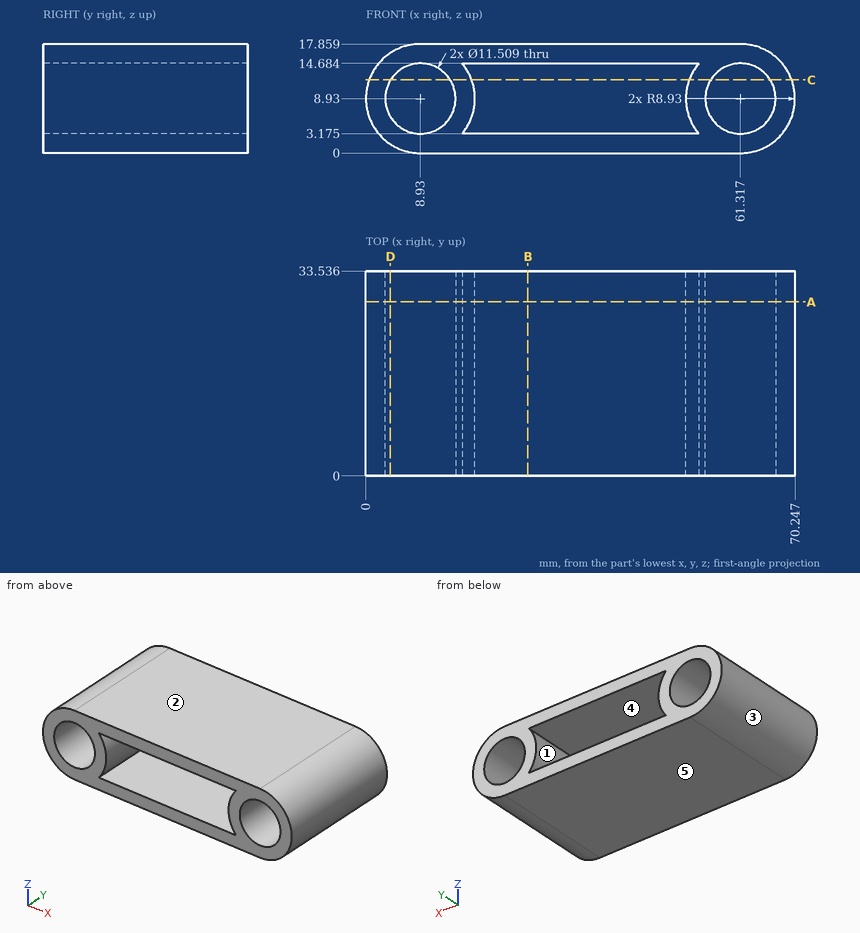
Geometry check sheet. Reference: drawing and pictorial views, mm from the part's lowest x, y, z. A direction names the side the tool comes from. Round coordinates to 2 decimals unless told otherwise and drop trailing zeros. Write each loop counter-clockwise with the first axis right and the second up, starting at its lowest first coordinate (ties: lowest second). Pieces come first, ordered by that corner, then holes.
1. Draft check along Z on the marked faces 1, 2 and 3. Enter one of: +Z half, -Z half, draft (parallel to the pull), parting line (faces both ways), or undercut.
2. Scan lines: L1, parallel to X at y = 16.5, z = 8.5 (1 decimal); L2, parallel to Z at x = 45, y = 4.5 (1 decimal); L3, parallel to X at y = 19, z = 8.75 (1 decimal). Record each from-to range of solid material in increasing order.
3. Section check C-C on z = 12. State how many separate pieces and enclosed holes the cut face has, plus the area to 3 significant figures.
4. Gauge pin test, flat ends, axial feed: P1, Ø5, axis at x = 36, z = 6.5, coming from the +Y side; P2, Ø2, axis at y = 9.5, z = 7.5, coming from the +X side; P3, Ø1.5, axis at x = 7.5, y = 13.5, coming from the +Z side. Record the tip position at first contact, or that the pin passes through.
5. Access from +Z, -Z, +X, -X, +Y, -Y to the whole of each face (thin tool, end or side, straight path). Record for the marked faces 4 and 5.
6. Section check A-A on y = 28.5. Enter the section's corners in (x, z) (1 decimal).
7. Section check D-D on x = 4. Enter the section's corners in (y, z) (1 decimal), plus the area to 3 significant figures.
8. Section check B-B on x = 26.5. Enter the section's corners in (y, z) (1 decimal), plus the area to 3 significant figures.
Answer:
1. face 1: undercut
1. face 2: +Z half
1. face 3: parting line
2. L1: x = 0 to 3.2, 14.7 to 17.8, 52.4 to 55.6, 67.1 to 70.2
2. L2: z = 0 to 3.2, 14.7 to 17.9
2. L3: x = 0 to 3.2, 14.7 to 17.9, 52.4 to 55.6, 67.1 to 70.2
3. separate pieces: 4
3. enclosed holes: 0
3. area: 472 mm2
4. P1: passes through
4. P2: stops at x = 70.24
4. P3: stops at z = 17.83
5. face 4: +Y, -Y
5. face 5: -Z, +X, -X, +Y, -Y
6. outline: (8.9, 0) - (61.3, 0) arc R8.9 ccw to (61.3, 17.9) - (8.9, 17.9) arc R8.9 ccw to start; hole circle Ø11.5 at (8.9, 8.9); hole (15.8, 3.2) - (54.5, 3.2) arc R8.9 cw to (54.5, 14.7) - (15.8, 14.7) arc R8.9 cw to start; hole circle Ø11.5 at (61.3, 8.9)
7. outline: (0, 1.5) - (33.5, 1.5) - (33.5, 6) - (0, 6) - close; (0, 11.9) - (33.5, 11.9) - (33.5, 16.4) - (0, 16.4) - close
7. area: 300 mm2
8. outline: (0, 0) - (33.5, 0) - (33.5, 3.2) - (0, 3.2) - close; (0, 14.7) - (33.5, 14.7) - (33.5, 17.9) - (0, 17.9) - close
8. area: 213 mm2
